```python
from build123d import *

# Parameters (mm, degrees)
F0_W     = 18
F0_H     = 14
F0_W_2   = 19
F0_H_2   = 16
F1_DEPTH = 2
F2_DEPTH = 14
F3_DEPTH = 16
F5_D     = 12.2
F7_D     = 12.2
F9_DEPTH = 25


# Not quite as in the source:
# - ends of sketch curves that miss each other by under 0.0002 mm in the source are joined


with BuildPart() as f1:
    # F0 (on Front) → F1 (new body)
    with BuildSketch(Plane.XZ):
        Polygon((9.5000003055, -25), (25, -25), (25, 25), (9.5000003055, 25), (9.5000003055, 8.9999977499), (-9.4999996945, 8.9999977499), (-9.4999996945, 24.9999977499), (-25, 25), (-25, -25), (-9.4999996945, -25), (-9.4999996945, -9), (9.5000003055, -9), align=None)
        Rectangle(F0_W, F0_H, mode=Mode.SUBTRACT)
        with Locations((3.055e-07, -17)):
            Rectangle(F0_W_2, F0_H_2)
        Polygon((9.5000003055, 8.9999977499), (9.5000003055, 24.9999977499), (-9.4999996945, 25), (-9.4999996945, 8.9999977499), align=None)
    extrude(amount=F1_DEPTH)

    # F0 (on Front) → F2 (join)
    with BuildSketch(Plane.XZ):
        Rectangle(F0_W, F0_H)
    extrude(amount=F2_DEPTH)

    # F0 (on Front) → F3 (join)
    with BuildSketch(Plane.XZ):
        with Locations((3.055e-07, -17)):
            Rectangle(F0_W_2, F0_H_2)
        Polygon((9.5000003055, 8.9999977499), (9.5000003055, 24.9999977499), (-9.4999996945, 25), (-9.4999996945, 8.9999977499), align=None)
    extrude(amount=F3_DEPTH)

    # F5 (through all)
    with Locations(Plane.YZ.offset(9.5000003055)):
        with Locations((-8.1, -17)):
            Hole(F5_D / 2)

    # F7 (through all)
    with Locations(Plane.YZ.offset(9.5000003055)):
        with Locations((-8.1, 16.9999977499)):
            Hole(F7_D / 2)

    # F8 (on face) → F9 (cut)
    with BuildSketch(Plane.YZ.offset(9)):
        with BuildLine():
            Line((-12.0000001043, -2.0710677001), (-10.5355339977, -3.5355338068))
            ThreePointArc((-10.5355339977, -3.5355338068), (-11.6193977653, -1.9134170539), (-12.0000001043, 1.212e-07))
            Line((-12.0000001043, 1.212e-07), (-12.0000001043, -2.0710677001))
        make_face()
        with BuildLine():
            ThreePointArc((-2.0000001043, 1.118e-07), (-2.3806024392, 1.9134172673), (-3.4644661888, 3.5355340081))
            ThreePointArc((-3.4644661888, 3.5355340081), (-5.0865829362, 4.6193977717), (-7.0000001043, 5.0000001118))
            ThreePointArc((-7.0000001043, 5.0000001118), (-8.9134172661, 4.6193977743), (-10.5355340102, 3.5355340177))
            ThreePointArc((-10.5355340102, 3.5355340177), (-11.6193977651, 1.9134172779), (-12.0000001043, 1.212e-07))
            ThreePointArc((-12.0000001043, 1.212e-07), (-11.6193977653, -1.9134170539), (-10.5355339977, -3.5355338068))
            ThreePointArc((-10.5355339977, -3.5355338068), (-8.9134172579, -4.6193975542), (-7.0000001043, -4.9999998882))
            ThreePointArc((-7.0000001043, -4.9999998882), (-5.0865829425, -4.6193975508), (-3.4644661984, -3.5355337942))
            ThreePointArc((-3.4644661984, -3.5355337942), (-2.3806024418, -1.9134170501), (-2.0000001043, 1.118e-07))
        make_face()
        with BuildLine():
            ThreePointArc((-12.0000001043, 1.212e-07), (-11.6193977651, 1.9134172779), (-10.5355340102, 3.5355340177))
            Line((-10.5355340102, 3.5355340177), (-12.0000001043, 2.0710679236))
            Line((-12.0000001043, 2.0710679236), (-12.0000001043, 1.212e-07))
        make_face()
        with BuildLine():
            ThreePointArc((-10.5355340102, 3.5355340177), (-8.9134172661, 4.6193977743), (-7.0000001043, 5.0000001118))
            Line((-7.0000001043, 5.0000001118), (-9.0710679162, 5.0000001118))
            Line((-9.0710679162, 5.0000001118), (-10.5355340102, 3.5355340177))
        make_face()
        with BuildLine():
            ThreePointArc((-7.0000001043, 5.0000001118), (-5.0865829362, 4.6193977717), (-3.4644661888, 3.5355340081))
            Line((-3.4644661888, 3.5355340081), (-4.9289322924, 5.0000001118))
            Line((-4.9289322924, 5.0000001118), (-7.0000001043, 5.0000001118))
        make_face()
        with BuildLine():
            Line((-3.4644661984, -3.5355337942), (-2.0000000522, -2.071067648))
            Line((-2.0000001043, -2.071067648), (-2.0000001043, 1.118e-07))
            ThreePointArc((-2.0000001043, 1.118e-07), (-2.3806024418, -1.9134170501), (-3.4644661984, -3.5355337942))
        make_face()
        with BuildLine():
            Line((-2.0000001043, 1.118e-07), (-2.0000001043, 2.0710678715))
            Line((-2.0000000522, 2.0710678715), (-3.4644661888, 3.5355340081))
            ThreePointArc((-3.4644661888, 3.5355340081), (-2.3806024392, 1.9134172673), (-2.0000001043, 1.118e-07))
        make_face()
        with BuildLine():
            Line((-4.9289322924, -4.9999998882), (-3.4644661984, -3.5355337942))
            ThreePointArc((-3.4644661984, -3.5355337942), (-5.0865829425, -4.6193975508), (-7.0000001043, -4.9999998882))
            Line((-7.0000001043, -4.9999998882), (-4.9289322924, -4.9999998882))
        make_face()
        with BuildLine():
            Line((-9.0710679162, -4.9999998882), (-7.0000001043, -4.9999998882))
            ThreePointArc((-7.0000001043, -4.9999998882), (-8.9134172579, -4.6193975542), (-10.5355339977, -3.5355338068))
            Line((-10.5355339977, -3.5355338068), (-9.0710679162, -4.9999998882))
        make_face()
    extrude(amount=-F9_DEPTH, mode=Mode.SUBTRACT)


solid = f1.part
```
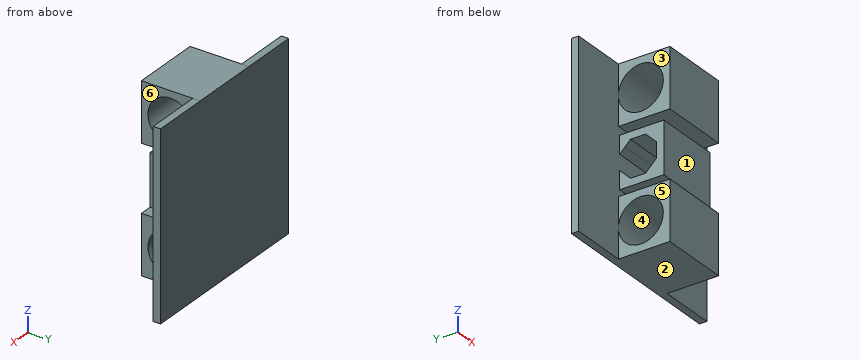
CAD build for the part. Positions are in the model's coordinates, mm. Face numbers are marked on the shaded views. A direction names the side the tool comes from. Round coordinates to 2 decimals unless told otherwise and drop trailing zeros. Loops run counter-clockwise (first coordinate to the right, second up) from the corner with the lowest first, then second, coordinate; pieces in that order, holes last. Notation, with made-up numbers: M 35,13 L 83,13 A25 ccw 83,28 Z; hole C 49.25,52.25 d6. An arc over 180 degrees is marked long. Use a Markdown table: item, result. Add a question column.
(1) Flat gauge pins, fed straight in: pin 1 (1.2 mm diameter, centred on x = 1, z = -1, fed in from +Y); pin 2 (7 mm diameter, centred on y = -7, z = -13, fed in from -X); pin 3 (2 mm diameter, centred on y = -13.5, z = 5.5, fed in from +X); pin 4 (9.5 mm diameter, centred on y = -10.5, z = 2, fed in from -X). Where does each tip first touch, or does it go through?
(2) Pull direction Z, two halves, no side cores. Call the marked faces 1, 2 and 3: +Z half, -Z half, draft (parallel to the pull), parting line (faces both ways), or undercut.
(3) Cut at C-C (y = -13.25). Give the cut face in (x, z).
(4) Drill centre lines: line 1 (Z direction, x = -1.25, y = -8.1); line 2 (Z direction, x = -3, y = -15.25); line 3 (Y direction, x = 3.5, z = -17). Where is each one in solid material? Low to high.
(5) Cut at B-B (y = -8.1). Give the cut face in (x, z).
(6) Cut at D-D (x = 15). Give the cut face in (y, z), and give its area (3 significant figures).
(7) Cut at A-A (z = -19). Give the cut face in (x, y).
(8) Which spindle directions (+Z, -Z, +X, -X, +Y, -Y) get a long thin tool onto all of the face, cutting with end or side? Do the marked faces 4, 5 and 6. Say none if no direction does.
Geometry says:
| question | item | result |
|---|---|---|
| 1 | pin 1 | stops at y = 0 |
| 1 | pin 2 | stops at x = -9.5 |
| 1 | pin 3 | stops at x = 9 |
| 1 | pin 4 | stops at x = -9 |
| 2 | face 1 | undercut |
| 2 | face 2 | -Z half |
| 2 | face 3 | draft |
| 3 | outline | M -9.5,-25 L 9.5,-25 L 9.5,-20.27 L -9.5,-20.27 Z; M -9.5,-13.73 L 9.5,-13.73 L 9.5,-9 L -9.5,-9 Z; M -9.5,9 L 9.5,9 L 9.5,13.73 L -9.5,13.73 Z; M -9.5,20.27 L 9.5,20.27 L 9.5,25 L -9.5,25 Z; M -9,-7 L 9,-7 L 9,7 L -9,7 Z |
| 4 | line 1 | z = -25 to -23.1, -10.9 to -9, -7 to -5, 5 to 7, 9 to 10.9, 23.1 to 25 |
| 4 | line 2 | z = -25 to -9, 9 to 25 |
| 4 | line 3 | y = -16 to -14.2, -2 to 0 |
| 5 | outline | M -9.5,-25 L 9.5,-25 L 9.5,-23.1 L -9.5,-23.1 Z; M -9.5,-10.9 L 9.5,-10.9 L 9.5,-9 L -9.5,-9 Z; M -9.5,9 L 9.5,9 L 9.5,10.9 L -9.5,10.9 Z; M -9.5,23.1 L 9.5,23.1 L 9.5,25 L -9.5,25 Z; M -9,-7 L 9,-7 L 9,-5 L -9,-5 Z; M -9,5 L 9,5 L 9,7 L -9,7 Z |
| 6 | outline | M -2,-25 L 0,-25 L 0,25 L -2,25 Z |
| 6 | area | 100 mm² |
| 7 | outline | M -25,-2 L -9.5,-2 L -9.5,-2.34 L 9.5,-2.34 L 9.5,-2 L 25,-2 L 25,0 L -25,0 Z; M -9.5,-16 L 9.5,-16 L 9.5,-13.86 L -9.5,-13.86 Z |
| 8 | face 4 | +X, -X |
| 8 | face 5 | +Z, -Z, -X, -Y |
| 8 | face 6 | +Z, -Z, +X, -Y |
